from build123d import *

# Parameters (mm, degrees)
BE_00_BOARD_DEPTH   = 0.381
SKETCH2_W           = 0.318200966
SKETCH2_H           = 0.54698776
SKETCH2_W_2         = 0.352186611
SKETCH2_H_2         = 0.526038031
BE_00_TRACES_DEPTH  = 0.022
BOSS_EXTRUDE1_DEPTH = 0.022


with BuildPart() as part:
    # Sketch1 → BE-00 Board (new body)
    with BuildSketch(Plane.XY):
        with BuildLine():
            Line((-8, 2.15), (-0.5, 2.15))
            ThreePointArc((-0.5, 2.15), (-0.146446609, 2.003553391), (0, 1.65))
            Line((0, 1.65), (0, -1.65))
            ThreePointArc((0, -1.65), (-0.146446609, -2.003553391), (-0.5, -2.15))
            Line((-0.5, -2.15), (-8, -2.15))
            ThreePointArc((-8, -2.15), (-8.353553391, -2.003553391), (-8.5, -1.65))
            Line((-8.5, -1.65), (-8.5, 1.65))
            ThreePointArc((-8.5, 1.65), (-8.353553391, 2.003553391), (-8, 2.15))
        make_face()
    extrude(amount=BE_00_BOARD_DEPTH)

    # Sketch2 → BE-00 Traces (add)
    with BuildSketch(Plane.XY.offset(0.381)):
        Polygon((-0.15, -0.17507), (-0.15, -0.32493), (-1.35, -0.57449), (-1.55024951, -0.70956), (-2.37, -0.70956), (-2.37, -0.28956), (-1.55024951, -0.28956), (-1.35, -0.42463), align=None)
        Polygon((-4.35, -0.56), (-7.35, -0.56), (-7.65, -0.516), (-8.35, -0.516), (-8.35, -0.754), (-7.65, -0.754), (-7.35, -0.71), (-4.35, -0.71), align=None)
        Polygon((-4.35, 0.71), (-4.35, 0.56), (-7.35, 0.56), (-7.65, 0.516), (-8.35, 0.516), (-8.35, 0.754), (-7.65, 0.754), (-7.35, 0.71), align=None)
        Polygon((-1.35, 0.42463), (-0.15, 0.17507), (-0.15, 0.32493), (-1.35, 0.57449), (-1.55024951, 0.70956), (-2.37, 0.70956), (-2.37, 0.28956), (-1.55024951, 0.28956), align=None)
        with Locations((-6.957835324, -1.501500363)):
            Rectangle(SKETCH2_W, SKETCH2_H)
        with Locations((-4.91735677, -1.316593308)):
            Rectangle(SKETCH2_W_2, SKETCH2_H_2)
    extrude(amount=BE_00_TRACES_DEPTH)

    # Sketch4 → Boss-Extrude1 (add)
    with BuildSketch(Plane(origin=(0, 0, 0), x_dir=(-1, 0, 0), z_dir=(0, 0, -1))):
        with BuildLine():
            Line((0.5, -2.05), (8, -2.05))
            ThreePointArc((8, -2.05), (8.282842712, -1.932842712), (8.4, -1.65))
            Line((8.4, -1.65), (8.4, 1.65))
            ThreePointArc((8.4, 1.65), (8.282842712, 1.932842712), (8, 2.05))
            Line((8, 2.05), (0.5, 2.05))
            ThreePointArc((0.5, 2.05), (0.217157288, 1.932842712), (0.1, 1.65))
            Line((0.1, 1.65), (0.1, -1.65))
            ThreePointArc((0.1, -1.65), (0.217157288, -1.932842712), (0.5, -2.05))
        make_face()
    extrude(amount=BOSS_EXTRUDE1_DEPTH)


solid = part.part
Could you check a few things on this model? Use its own coordinates, in mm. Give positions to 0.01 mm unless a question says otherwise; leave off trailing zeros. Answer as CSV lines item,"result". Start each with the question number.
(1) We'd pull the mould along Y, two halves only. Please class faces 1 (the flat face through (-4, 0, 0.381)), 2 (the flat face through (-4, 0, -0.022)): released by +Y, released by -Y, zero draft, split by the parting line, or undercut.
(2) I need wall thicknesses on probe 1 along Z at (x, y) = (-5.75, -0.15); probe 2 along X at (y, z) = (1.85, 0.15). Which ranges of each line are inside material? Lowest first, please.
(3) I'm going to push a flat-ended pin straight in: pin 1 Ø1.5 at (x, y) = (-3, -1.5) entering from +Z. Where does the tip first touch, or does it pass through?
Computed:
1,face 1,"undercut"
1,face 2,"zero draft"
2,probe 1,"z = -0.02 to 0.38"
2,probe 2,"x = -8.46 to -0.04"
3,pin 1,"stops at z = 0.38"
